The listing builds one solid part. Answer for the finished solid, in the listing's coordinates (mm). A direction names the side the tool comes from. Give positions to 0.01 mm unless a question says otherwise; leave off trailing zeros. Order: outer loops, then holes, each group sorted by start corner. A loop starts at its lowest first (then second) coordinate and runs counter-clockwise, first axis right, second up. Notation, with made-up numbers: (8.5, 62) - (17.5, 62) arc R28 ccw to (17.5, 85) - close; hole circle Ø5 at (9, -31.5). An arc over 180 degrees is marked (long way). Write each question's results on one line, items separated by ' | '. Start each with the question number.
1. Which of the six approach directions +Z, -Z, +X, -X, +Y, -Y give full straight-line access (tool end or side, diameter ignored) to faces 1 (the face through (680, 0, 11)), 2 (the face through (664, 0, 13))?
2. Find the intervals of material crossed by L1, parallel to Y at x = 240, z = 6.5; L2, parallel to Y at x = 660, z = 4.5; L3, parallel to Y at x = 496.5, z = 11.75, in increasing order.
3. Flat-ended cylindrical pins translate along their axes: pin 1 (5.5 mm diameter, centred on x = 480, y = 2.5, fed in from +Z); pin 2 (8 mm diameter, centred on x = 176.5, z = 11.5, fed in from +Y); pin 3 (2.5 mm diameter, centred on x = 267.5, z = 11.5, fed in from +Y). Find the tip coordinate at first contact, or state that the pin passes through.
4. Section A-A (x = 372.5) is taken. Give the vertices of the cut face in (y, z), and give its area (3 significant figures).
5. Determine the mould class of faces 3 (the face through (325, 0, 21.9)), 4 (the face through (-1.19, -5.37, 17.51)) for opening direction Y: released by +Y, released by -Y, zero draft, split by the parting line, or undercut.
from build123d import *

# Parameters (mm, degrees)
BOSS_EXTRUDE1_DEPTH                     = 700
SKETCH2_W                               = 700
SKETCH2_H                               = 9.898648987
BOSS_EXTRUDE2_DEPTH                     = 3.8
SKETCH3_W                               = 700
SKETCH3_H                               = 6.0986495
BOSS_EXTRUDE3_DEPTH                     = 3.8
CUT_EXTRUDE1_DEPTH                      = 701.436906509
CUT_EXTRUDE2_DEPTH                      = 701.436906509
DRAFT1_ANGLE                            = 44.999996129
DRAFT2_ANGLE                            = 44.999996129
CBORE_FOR_M6_HEX_HEAD_BOLT1_D           = 7
CBORE_FOR_M6_HEX_HEAD_BOLT1_CBORE_D     = 11
CBORE_FOR_M6_HEX_HEAD_BOLT1_CBORE_DEPTH = 8.9
CHAMFER1_SIZE                           = 0.184878832
CHAMFER1_SIZE_2                         = 0.188416661
CHAMFER2_SIZE                           = 0.377828878
CHAMFER2_SIZE_2                         = 0.356334292
CHAMFER3_SIZE                           = 1.5


with BuildPart() as part:
    # Sketch1 → Boss-Extrude1 (new body)
    with BuildSketch(Plane(origin=(-20, 0, 0), x_dir=(0, -1, 0), z_dir=(-1, 0, 0))):
        with BuildLine():
            Line((-7.7, 0), (7.7, 0))
            Line((7.7, 0), (7.7, 13.280138132))
            Line((7.7, 13.280138132), (8.929704991, 14.509842724))
            ThreePointArc((8.929704991, 14.509842724), (9.732349977, 16.117560007), (11.4, 16.786841141))
            Line((11.4, 16.786841141), (11.4, 21.9))
            Line((11.4, 21.9), (-11.4, 21.9))
            Line((-11.4, 21.9), (-11.4, 16.786841141))
            ThreePointArc((-11.4, 16.786841141), (-9.732349977, 16.117560007), (-8.929704991, 14.509842724))
            Line((-8.929704991, 14.509842724), (-7.7, 13.280138132))
            Line((-7.7, 13.280138132), (-7.7, 0))
        make_face()
    extrude(amount=-BOSS_EXTRUDE1_DEPTH)

    # Sketch2 → Boss-Extrude2 (add)
    with BuildSketch(Plane.XZ.offset(7.7)):
        with Locations((330, 4.949324494)):
            Rectangle(SKETCH2_W, SKETCH2_H)
    extrude(amount=BOSS_EXTRUDE2_DEPTH)

    # Sketch3 → Boss-Extrude3 (add)
    with BuildSketch(Plane(origin=(0, 7.7, 0), x_dir=(-1, 0, 0), z_dir=(0, 1, 0))):
        with Locations((-330, 3.04932475)):
            Rectangle(SKETCH3_W, SKETCH3_H)
    extrude(amount=BOSS_EXTRUDE3_DEPTH)

    # Sketch4 → Cut-Extrude1 (cut, through all)
    with BuildSketch(Plane(origin=(680, 0, 0), x_dir=(0, 0, -1), z_dir=(1, 0, 0))):
        with BuildLine():
            Line((-21.9, -11.4), (-19.212914859, -11.4))
            ThreePointArc((-19.212914859, -11.4), (-20.027311235, -9.587199721), (-21.9, -8.921975628))
            Line((-21.9, -8.921975628), (-21.9, -11.4))
        make_face()
    extrude(amount=-CUT_EXTRUDE1_DEPTH, mode=Mode.SUBTRACT)

    # Sketch5 → Cut-Extrude2 (cut, through all)
    with BuildSketch(Plane(origin=(680, 0, 0), x_dir=(0, 0, -1), z_dir=(1, 0, 0))):
        with BuildLine():
            Line((-21.9, 11.4), (-21.9, 8.921975628))
            ThreePointArc((-21.9, 8.921975628), (-20.027311235, 9.587199721), (-19.212914859, 11.4))
            Line((-19.212914859, 11.4), (-21.9, 11.4))
        make_face()
    extrude(amount=-CUT_EXTRUDE2_DEPTH, mode=Mode.SUBTRACT)

    # Draft1
    draft1_faces = [part.faces().sort_by_distance(p)[0] for p in [
        (330, 9.6, 6.0986495),
    ]]
    draft(draft1_faces, Plane.ZX.offset(11.5), DRAFT1_ANGLE)

    # Draft2
    draft2_faces = [part.faces().sort_by_distance(p)[0] for p in [
        (330, -9.6, 9.898648987),
    ]]
    draft(draft2_faces, Plane(origin=(680, -7.7, 0), x_dir=(0, 0, -1), z_dir=(0, -1, 0)), DRAFT2_ANGLE)

    # CBORE for M6 Hex Head Bolt1 (through all)
    with Locations(Plane.XY.offset(21.9)):
        with Locations((60, 0), (120, 0), (180, 0), (240, 0), (300, 0), (360, 0), (420, 0), (480, 0), (540, 0), (600, 0), (660, 0), (0, 0)):
            CounterBoreHole(CBORE_FOR_M6_HEX_HEAD_BOLT1_D / 2, CBORE_FOR_M6_HEX_HEAD_BOLT1_CBORE_D / 2, CBORE_FOR_M6_HEX_HEAD_BOLT1_CBORE_DEPTH)

    # Chamfer1
    # the kernel refuses this chamfer: 0.188416661, 0.184878832 mm, written as the material it takes off along each edge
    with BuildSketch(Plane(origin=(-20.505430952, 11.4, 16.786841141), x_dir=(0, -0.9983504789140061, -0.057413598146908586), z_dir=(1, 0, 0))) as chamfer1_piece_1:
        with BuildLine():
            Line((0.196483777, 0), (-CHAMFER1_SIZE * 0.0574135982779, -CHAMFER1_SIZE * 0.998350481192))
            Line((-CHAMFER1_SIZE * 0.0574135982779, -CHAMFER1_SIZE * 0.998350481192), (0, 0))
            ThreePointArc((0, 0), (0.101060009, -0.001906555), (0.196483777, 0))
        make_face()
    extrude(amount=701.010861905, mode=Mode.SUBTRACT)
    with BuildSketch(Plane(origin=(680.505430952, 11.4, 19.212914859), x_dir=(0, 0, -1), z_dir=(-1, 0, 0))) as chamfer1_piece_2:
        with BuildLine():
            Line((CHAMFER1_SIZE * 1.00000000228, 0), (-0.011280841, 0.196159673))
            ThreePointArc((-0.011280841, 0.196159673), (-0.003898809, 0.10100277), (0, 0))
            Line((0, 0), (CHAMFER1_SIZE * 1.00000000228, 0))
        make_face()
    extrude(amount=701.010861905, mode=Mode.SUBTRACT)
    with BuildSketch(Plane(origin=(-20.49480589, -11.4, 16.786841141), x_dir=(0, 0, 1), z_dir=(1, 0, 0))) as chamfer1_piece_3:
        with BuildLine():
            Line((CHAMFER1_SIZE_2 * 1.0000000015, 0), (-0.010884434, -0.192019871))
            ThreePointArc((-0.010884434, -0.192019871), (-0.003775118, -0.098877649), (0, 0))
            Line((0, 0), (CHAMFER1_SIZE_2 * 1.0000000015, 0))
        make_face()
    extrude(amount=700.98961178, mode=Mode.SUBTRACT)
    with BuildSketch(Plane(origin=(680.49480589, -11.4, 19.212914859), x_dir=(0, 0.9983973290920217, 0.05659304959018505), z_dir=(-1, 0, 0))) as chamfer1_piece_4:
        with BuildLine():
            Line((0.19232811, 0), (-CHAMFER1_SIZE_2 * 0.0565930496749, CHAMFER1_SIZE_2 * 0.998397330587))
            Line((-CHAMFER1_SIZE_2 * 0.0565930496749, CHAMFER1_SIZE_2 * 0.998397330587), (0, 0))
            ThreePointArc((0, 0), (0.098932826, 0.00182672), (0.19232811, 0))
        make_face()
    extrude(amount=700.98961178, mode=Mode.SUBTRACT)

    # Chamfer2
    # the kernel refuses this chamfer: 0.377828878, 0.356334292 mm, written as the material it takes off along each edge
    with BuildSketch(Plane(origin=(680.984980067, -8.921975628, 21.9), x_dir=(0, 1, 0), z_dir=(-1, 0, 0))) as chamfer2_piece_1:
        with BuildLine():
            Line((CHAMFER2_SIZE, 0), (-0.005157634, 0.382986696))
            ThreePointArc((-0.005157634, 0.382986696), (0.004600101, 0.197032231), (0, 0))
            Line((0, 0), (CHAMFER2_SIZE, 0))
        make_face()
    extrude(amount=701.969960134, mode=Mode.SUBTRACT)
    with BuildSketch(Plane(origin=(681.061335524, 8.921975628, 21.9), x_dir=(0, 0.01938777487044788, -0.9998120394281981), z_dir=(-1, 0, 0))) as chamfer2_piece_2:
        with BuildLine():
            Line((0.412898561, 0), (-CHAMFER2_SIZE_2 * 0.0193877748633, CHAMFER2_SIZE_2 * 0.999812039061))
            Line((-CHAMFER2_SIZE_2 * 0.0193877748633, CHAMFER2_SIZE_2 * 0.999812039061), (0, 0))
            ThreePointArc((0, 0), (0.212241278, 0.008430622), (0.412898561, 0))
        make_face()
    extrude(amount=702.122671049, mode=Mode.SUBTRACT)

    # Chamfer3
    chamfer3_edges = [part.edges().sort_by_distance(p)[0] for p in [
        (330, -11.5, 0),
        (330, 11.5, 0),
    ]]
    chamfer(chamfer3_edges, length=CHAMFER3_SIZE)


solid = part.part
Reported:
1) face 1: +Z, -Z, +X, +Y, -Y | face 2: +Z
2) L1: -11.1 to -3.5, 3.5 to 11.1 | L2: -11.5 to -3.5, 3.5 to 11.5 | L3: -7.7 to 7.7
3) pin 1: z = 13 | pin 2: y = 10.1 | pin 3: y = 7.7
4) outline: (-11.5, 1.5) - (-10, 0) - (10, 0) - (11.5, 1.5) - (11.5, 6.1) - (7.7, 9.9) - (7.7, 13.28) - (8.93, 14.51) arc R2.53 cw to (11.2, 16.78) - (11.4, 16.97) - (11.4, 19.03) - (11.2, 19.22) arc R2.53 cw to (8.93, 21.49) - (8.57, 21.9) - (-8.54, 21.9) - (-8.93, 21.52) arc R2.53 cw to (-11.21, 19.22) - (-11.4, 19.02) - (-11.4, 16.98) - (-11.21, 16.78) arc R2.53 cw to (-8.93, 14.51) - (-7.7, 13.28) - (-7.7, 9.9) - (-11.5, 6.1) - close | area: 433 mm²
5) face 3: zero draft | face 4: undercut
